from build123d import *

# Parameters (mm, degrees)
BOSS_EXTRUDE1_DEPTH = 25.4
CUT_EXTRUDE1_DEPTH  = 25.4
CUT_EXTRUDE2_DEPTH  = 25.4
SKETCH4_R           = 18.8
CUT_EXTRUDE3_DEPTH  = 25.4


with BuildPart() as part:
    # Sketch1 → Boss-Extrude1 (new body)
    with BuildSketch(Plane.XY):
        Polygon((0, 21), (21, 21), (21, -21), (-21, -21), (-21, 21), align=None)
    extrude(amount=BOSS_EXTRUDE1_DEPTH)

    # Sketch2 → Cut-Extrude1 (cut)
    with BuildSketch(Plane.XY.offset(25.4)):
        Polygon((21, 21), (21, 14), (16, 14), (14, 16), (14, 21), align=None)
    extrude(amount=-CUT_EXTRUDE1_DEPTH, mode=Mode.SUBTRACT)

    # Sketch3 → Cut-Extrude2 (cut)
    with BuildSketch(Plane.XY.offset(25.4)):
        Polygon((-14, -16), (-16, -14), (-21, -14), (-21, -21), (-14, -21), align=None)
    extrude(amount=-CUT_EXTRUDE2_DEPTH, mode=Mode.SUBTRACT)

    # Sketch4 → Cut-Extrude3 (cut)
    with BuildSketch(Plane.XY.offset(25.4)):
        Circle(SKETCH4_R)
    extrude(amount=-CUT_EXTRUDE3_DEPTH, mode=Mode.SUBTRACT)


solid = part.part
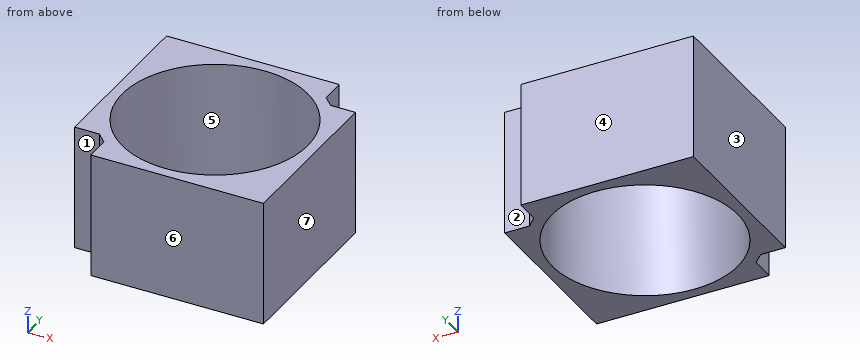
Source: CAD feature listing. Evaluate the final solid. Frame: model axes, mm. Face numbers are marked on the shaded views. A direction names the side the tool comes from. Coordinates: 2 decimals unless noted, no trailing zeros. Loops run counter-clockwise (first coordinate to the right, second up) from the corner with the lowest first, then second, coordinate; pieces in that order, holes last. Notation, with made-up numbers: (18, -16.5) - (57, -16.5) arc R24 cw to (57, 11.5) - close; hole circle Ø9 at (83, 32.25). An arc over 180 degrees is marked (long way). Return JSON: item names as keys, results as strings.
Q1. Access query for the marked faces 1, 2 and 3. Directions: +Z, -Z, +X, -X, +Y, -Y. A direction counts if a zero-diameter tool reaches every point of the face in a straight line with its end or side. Return the directions, or none.
Results:
{"face 1": "+Z, -Z, -X, -Y", "face 2": "+Z, -Z, +X, +Y", "face 3": "+Z, -Z, -X, +Y, -Y"}
Q2. Section A-A, the plane y = 0. Return loops of the section in (x, z), plus the area to 3 significant figures.
Results:
{"outline": "(-21, 0) - (-18.8, 0) - (-18.8, 25.4) - (-21, 25.4) - close; (18.8, 0) - (21, 0) - (21, 25.4) - (18.8, 25.4) - close", "area": "112 mm2"}
Q3. Mould query, pull axis Y, two halves, no side actions, for the marked faces 4, 5, 6 and 7. Classes: released by +Y, released by -Y, zero draft, split by the parting line, or undercut.
Results:
{"face 4": "released by +Y", "face 5": "undercut", "face 6": "released by -Y", "face 7": "zero draft"}
Q4. Material intervals for line 1 along Y through (x, z) = (0, 10.5); line 2 along Y through (x, z) = (-17, 17); line 3 along X through (y, z) = (6, 9.75), sorted ascending.
Results:
{"line 1": "-21 to -18.8, 18.8 to 21", "line 2": "-14 to -8.03, 8.03 to 21", "line 3": "-21 to -17.82, 17.82 to 21"}
Q5. Contact query for flat-ended pins moving along their axis: P1, Ø3, axis at y = 16, z = 4, coming from the +X side; P2, Ø10, axis at y = -15, z = 7, coming from the -X side; P3, Ø2.5, axis at y = -17.5, z = 8, coming from the -X side; P4, Ø2.5, axis at x = 18, z = 18.5, coming from the +Y side. Output: stop coordinate, or through.
Results:
{"P1": "x = 15.5", "P2": "x = -21", "P3": "x = -14", "P4": "y = 14"}
Q6. Section C-C, the plane z = 4.75. Return loops of the section in (x, y), plus the area to 3 significant figures.
Results:
{"outline": "(-21, -14) - (-16, -14) - (-14, -16) - (-14, -21) - (21, -21) - (21, 14) - (16, 14) - (14, 16) - (14, 21) - (-21, 21) - close; hole circle Ø37.6 at (0, 0)", "area": "560 mm2"}
